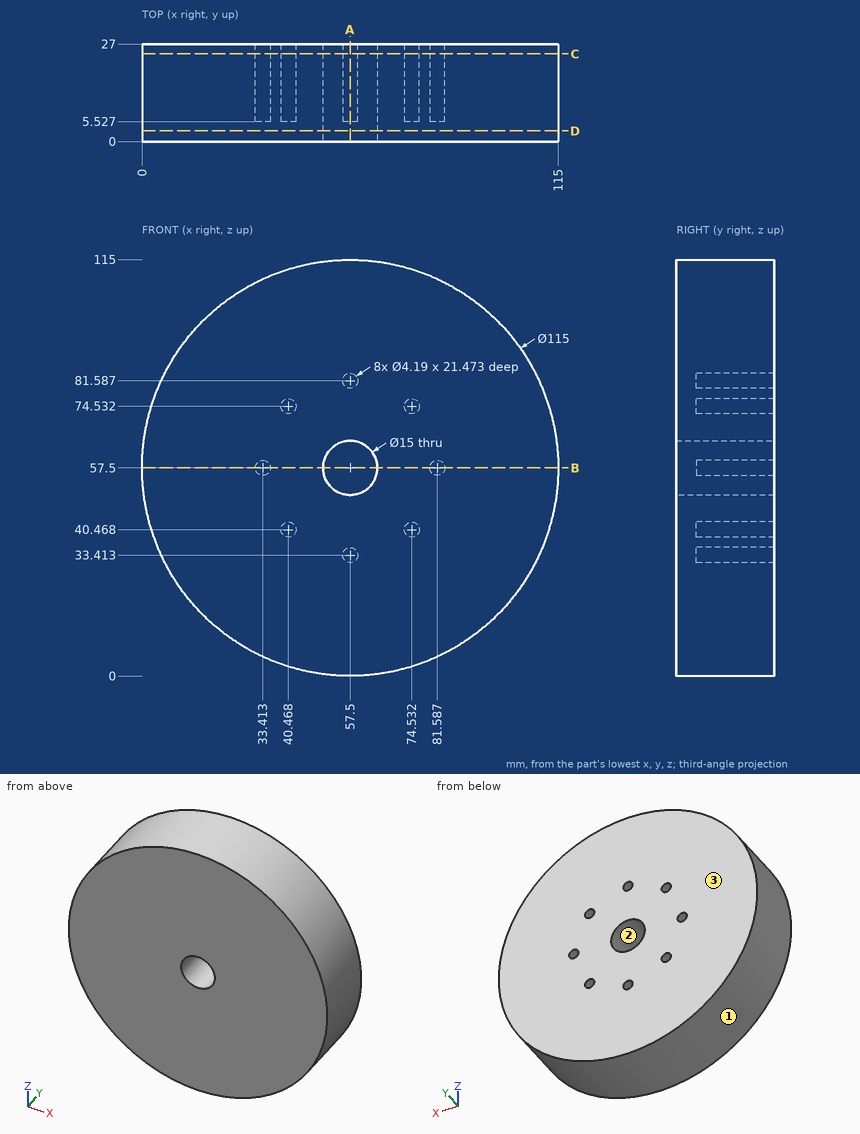
For this review, use the dimensioned drawing (mm, ordinates from the lowest corner) and the shaded views. Give positions to 0.01 mm unless a question says otherwise; leave off trailing zeros. Loops run counter-clockwise (first coordinate to the right, second up) from the corner with the lowest first, then second, coordinate; pieces in that order, holes last.
Item 1: Take a section at C-C, the plane y = 24.25. Give the number of separate pieces and of enclosed holes in the cut face, and give its area (3 significant figures).
Item 2: Take a section at B-B, the plane z = 57.5. State the section outline as (x, y) points.
Item 3: Take a section at D-D, the plane y = 3. State the section outline as (x, z) points.
Item 4: Insertion check: pin 1 (12 mm diameter, centred on y = 23.5, z = 69, fed in from -X); pin 2 (10 mm diameter, centred on x = 28, y = 22.5, fed in from +Z); pin 3 (1.3 mm diameter, centred on x = 58, z = 81.5, fed in from +Y). Each pin has a flat end and moves straight along its axis. Give the tip position at first contact, or say it passes through.
Item 5: For line 1 along X through (y, z) = (18.75, 57.5); line 2 along X through (y, z) = (14.75, 41) (1 decimal); line 3 along Z through (x, y) = (61.5, 22.5) (1 decimal), list the stretches that pass through material, from the lowest coordinate up.
Item 6: Take a section at A-A, the plane x = 57.5. State the section outline as (y, z) points.
Item 7: Draft analysis for pull direction Z (two halves, no side actions). For the marked faces 1, 2 and 3, state which applies: +Z half, -Z half, draft (parallel to the pull), parting line (faces both ways), or undercut.
Calculated:
1. separate pieces: 1
1. enclosed holes: 9
1. area: 10,100 mm2
2. outline: (0, 0) - (50, 0) - (50, 27) - (35.51, 27) - (35.51, 5.53) - (31.32, 5.53) - (31.32, 27) - (0, 27) - close; (65, 0) - (115, 0) - (115, 27) - (83.68, 27) - (83.68, 5.53) - (79.49, 5.53) - (79.49, 27) - (65, 27) - close
3. outline: circle Ø115 at (57.5, 57.5); hole circle Ø15 at (57.5, 57.5)
4. pin 1: stops at x = 0.26
4. pin 2: stops at z = 109.52
4. pin 3: stops at y = 5.53
5. line 1: x = 0 to 31.32, 35.51 to 50, 65 to 79.49, 83.68 to 115
5. line 2: x = 2.4 to 38.4, 42.5 to 72.5, 76.6 to 112.6
5. line 3: z = 0.1 to 51.2, 63.8 to 114.9
6. outline: (0, 0) - (27, 0) - (27, 31.32) - (5.53, 31.32) - (5.53, 35.51) - (27, 35.51) - (27, 50) - (0, 50) - close; (0, 65) - (27, 65) - (27, 79.49) - (5.53, 79.49) - (5.53, 83.68) - (27, 83.68) - (27, 115) - (0, 115) - close
7. face 1: parting line
7. face 2: undercut
7. face 3: draft
